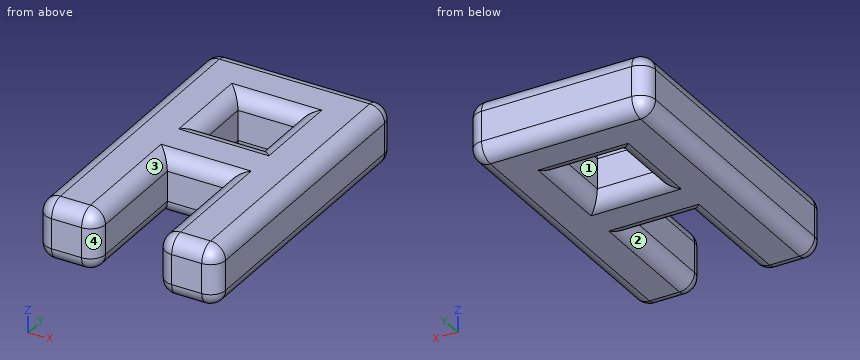
```python
from build123d import *

# Parameters (mm, degrees)
F0_W     = 15.24
F0_H     = 25.4
F1_DEPTH = 5.08
F2_W     = 5.08
F2_H     = 5.08
F2_H_2   = 10.16
F3_DEPTH = 5.08
F4_R     = 1.27


with BuildPart() as f1:
    # F0 (on Top) → F1 (new body)
    with BuildSketch(Plane.XY):
        Rectangle(F0_W, F0_H)
    extrude(amount=F1_DEPTH)

    # F2 (on face) → F3 (cut)
    with BuildSketch(Plane.XY.offset(5.08)):
        with Locations((0, 5.08)):
            Rectangle(F2_W, F2_H)
        with Locations((0, -7.62)):
            Rectangle(F2_W, F2_H_2)
    extrude(amount=-F3_DEPTH, mode=Mode.SUBTRACT)

    # F4
    f4_edges = [f1.edges().sort_by_distance(p)[0] for p in [
        (-7.62, 12.7, 2.54),
        (-7.62, -12.7, 2.54),
        (0, 2.54, 5.08),
        (2.54, 5.08, 5.08),
        (-2.54, 5.08, 5.08),
        (0, 7.62, 5.08),
        (0, 12.7, 5.08),
        (0, 12.7, 0),
        (7.62, 12.7, 2.54),
        (0, -2.54, 5.08),
        (0, -2.54, 0),
        (2.54, -7.62, 5.08),
        (-2.54, -7.62, 5.08),
        (7.62, 0, 0),
        (7.62, 0, 5.08),
        (7.62, -12.7, 2.54),
        (5.08, -12.7, 5.08),
        (5.08, -12.7, 0),
        (2.54, -12.7, 2.54),
        (-5.08, -12.7, 5.08),
        (-2.54, -12.7, 2.54),
        (-7.62, 0, 5.08),
        (-5.08, -12.7, 0),
        (0, 2.54, 0),
        (-2.54, 5.08, 0),
        (0, 7.62, 0),
        (2.54, 5.08, 0),
        (-7.62, 0, 0),
        (-2.54, -7.62, 0),
        (2.54, -7.62, 0),
    ]]
    fillet(f4_edges, radius=F4_R)


solid = f1.part
```
Input: part model. Units: mm. Frame: model coordinates. Face numbers are marked on the shaded views. A direction names the side the tool comes from. Give positions to 0.01 mm unless a question says otherwise; leave off trailing zeros. Order: outer loops, then holes, each group sorted by start corner. A loop starts at its lowest first (then second) coordinate and runs counter-clockwise, first axis right, second up. Notation, with made-up numbers: (-8.75, 48) - (32.25, 48) arc R16 cw to (32.25, 64) - close; hole circle Ø6 at (21, 38). An arc over 180 degrees is marked (long way). Use a Markdown table: item, result.
(1) Access query for the marked faces 1, 2, 3 and 4. Directions: +Z, -Z, +X, -X, +Y, -Y. A direction counts if a zero-diameter tool reaches every point of the face in a straight line with its end or side. Return the directions, or none.
Computed values:
| item | result |
|---|---|
| face 1 | +Z, -Z |
| face 2 | -Z, -Y |
| face 3 | +Z, -Y |
| face 4 | +Z, -Z, -Y |
(2) Section query B-B (y = -8.5). Output: boundary loops of the cut face in (x, z), then the cut area to 3 significant figures.
Computed values:
| item | result |
|---|---|
| outline | (-7.62, 1.27) arc R1.27 ccw to (-6.35, 0) - (-3.81, 0) arc R1.27 ccw to (-2.54, 1.27) - (-2.54, 3.81) arc R1.27 ccw to (-3.81, 5.08) - (-6.35, 5.08) arc R1.27 ccw to (-7.62, 3.81) - close; (2.54, 1.27) arc R1.27 ccw to (3.81, 0) - (6.35, 0) arc R1.27 ccw to (7.62, 1.27) - (7.62, 3.81) arc R1.27 ccw to (6.35, 5.08) - (3.81, 5.08) arc R1.27 ccw to (2.54, 3.81) - close |
| area | 48.8 mm2 |
(3) Section query C-C (z = 2.55). Output: boundary loops of the cut face in (x, y), then the cut area to 3 significant figures.
Computed values:
| item | result |
|---|---|
| outline | (-7.62, -11.43) arc R1.27 ccw to (-6.35, -12.7) - (-3.81, -12.7) arc R1.27 ccw to (-2.54, -11.43) - (-2.54, -2.54) - (2.54, -2.54) - (2.54, -11.43) arc R1.27 ccw to (3.81, -12.7) - (6.35, -12.7) arc R1.27 ccw to (7.62, -11.43) - (7.62, 11.43) arc R1.27 ccw to (6.35, 12.7) - (-6.35, 12.7) arc R1.27 ccw to (-7.62, 11.43) - close; hole (-2.54, 2.54) - (2.54, 2.54) - (2.54, 7.62) - (-2.54, 7.62) - close |
| area | 308 mm2 |
(4) Section query A-A (x = 0.25). Output: boundary loops of the cut face in (y, z), then the cut area to 3 significant figures.
Computed values:
| item | result |
|---|---|
| outline | (-2.54, 1.27) arc R1.27 ccw to (-1.27, 0) - (1.27, 0) arc R1.27 ccw to (2.54, 1.27) - (2.54, 3.81) arc R1.27 ccw to (1.27, 5.08) - (-1.27, 5.08) arc R1.27 ccw to (-2.54, 3.81) - close; (7.62, 1.27) arc R1.27 ccw to (8.89, 0) - (11.43, 0) arc R1.27 ccw to (12.7, 1.27) - (12.7, 3.81) arc R1.27 ccw to (11.43, 5.08) - (8.89, 5.08) arc R1.27 ccw to (7.62, 3.81) - close |
| area | 48.8 mm2 |
(5) Line query: line 1 (X direction, y = -6.25, z = 1.9); line 2 (Y direction, x = -1, z = 3.4); line 3 (Y direction, x = -2.25, z = 0.5). Output: solid intervals per line, ascending. Write a range as from..to.
Computed values:
| item | result |
|---|---|
| line 1 | x = -7.62..-2.54, 2.54..7.62 |
| line 2 | y = -2.54..2.54, 7.62..12.7 |
| line 3 | y = -2.28..2.28, 7.88..12.44 |
(6) Pin query (flat end, axial travel): pin 1 (3 mm diameter, centred on x = 0.5, z = 3, fed in from -Y). Return the tip coordinate at first contact, or that it passes through.
Computed values:
| item | result |
|---|---|
| pin 1 | stops at y = -2.54 |
(7) Section query D-D (y = 9.75). Output: boundary loops of the cut face in (x, z).
Computed values:
| item | result |
|---|---|
| outline | (-7.62, 1.27) arc R1.27 ccw to (-6.35, 0) - (6.35, 0) arc R1.27 ccw to (7.62, 1.27) - (7.62, 3.81) arc R1.27 ccw to (6.35, 5.08) - (-6.35, 5.08) arc R1.27 ccw to (-7.62, 3.81) - close |
